from build123d import *

# Parameters (mm, degrees)
CROQUIS1_W              = 25
CROQUIS1_H              = 23
SALIENTE_EXTRUIR1_DEPTH = 2
CROQUIS2_W              = 8.5
CROQUIS2_H              = 8.5
SALIENTE_EXTRUIR2_DEPTH = 3
CROQUIS3_R              = 3.75
SALIENTE_EXTRUIR3_DEPTH = 3
CROQUIS4_R              = 0.875
CORTAR_EXTRUIR1_DEPTH   = 3
CROQUIS5_W              = 22
CROQUIS5_H              = 5.5
SALIENTE_EXTRUIR4_DEPTH = 2


with BuildPart() as part:
    # Croquis1 → Saliente-Extruir1 (new body)
    with BuildSketch(Plane(origin=(0, 0, 0), x_dir=(1, 0, 0), z_dir=(0, 1, 0))):
        Rectangle(CROQUIS1_W, CROQUIS1_H)
    extrude(amount=SALIENTE_EXTRUIR1_DEPTH)

    # Croquis2 → Saliente-Extruir2 (add)
    with BuildSketch(Plane.XZ):
        with Locations((0, -1.75)):
            Rectangle(CROQUIS2_W, CROQUIS2_H)
    extrude(amount=SALIENTE_EXTRUIR2_DEPTH)

    # Croquis3 → Saliente-Extruir3 (add)
    with BuildSketch(Plane.XZ.offset(3)):
        with Locations((0, -1.75)):
            Circle(CROQUIS3_R)
    extrude(amount=SALIENTE_EXTRUIR3_DEPTH)

    # Croquis4 → Cortar-Extruir1 (cut)
    with BuildSketch(Plane.XZ):
        with Locations((-10.625, 9.625)):
            Circle(CROQUIS4_R)
        with Locations((10.825, 9.625)):
            Circle(CROQUIS4_R)
        with Locations((10.825, -3.375)):
            Circle(CROQUIS4_R)
        with Locations((-10.625, -3.375)):
            Circle(CROQUIS4_R)
    extrude(amount=-CORTAR_EXTRUIR1_DEPTH, mode=Mode.SUBTRACT)

    # Croquis5 → Saliente-Extruir4 (add)
    with BuildSketch(Plane(origin=(0, 2, 0), x_dir=(1, 0, 0), z_dir=(0, 1, 0))):
        with Locations((0, 9.75)):
            Rectangle(CROQUIS5_W, CROQUIS5_H)
    extrude(amount=SALIENTE_EXTRUIR4_DEPTH)


solid = part.part
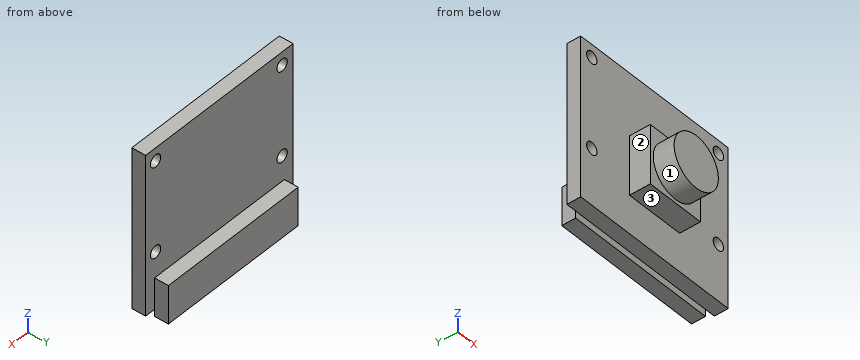
Model file for the job. Use its own axes, mm. Face numbers are marked on the shaded views. A direction names the side the tool comes from. Give positions to 0.01 mm unless a question says otherwise; leave off trailing zeros. Loops run counter-clockwise (first coordinate to the right, second up) from the corner with the lowest first, then second, coordinate; pieces in that order, holes last.
1) Wall check: line 1 (X direction, y = 1.25, z = -3); line 2 (Z direction, x = -6, y = 2.5); line 3 (Y direction, x = -3, z = 9). Give the ranges that are in metal, low to high.
2) Saw through at B-B (y = 0.75). Write the cut outline in (x, z) (3 decimals), plus the area to 3 significant figures.
3) Saw through at C-C (x = 0). Write the cut outline in (y, z).
4) Tool access for the marked faces 1, 2 and 3: list every direction of +Z, -Z, +X, -X, +Y, -Y with a clear straight run to the whole face (end or side of a thin tool).
5) Flat gauge pins, fed straight in: pin 1 Ø1.6 at (x, z) = (-10.625, -3.375) entering from -Y; pin 2 Ø3 at (x, z) = (10.825, 9.625) entering from -Y; pin 3 Ø0.9 at (x, y) = (-0.5, -1) entering from -Z; pin 4 Ø0.6 at (x, y) = (5, 1.5) entering from -Z. Where does each tip first touch, or does it go through?
6) Saw through at D-D (y = 2.5). Write the cut outline in (x, z).
7) Saw through at A-A (z = -1.75). Write the cut outline in (x, y), plus the area to 3 significant figures.
Answer block:
1. line 1: x = -12.5 to -11.42, -9.83 to 10.03, 11.62 to 12.5
1. line 2: z = -12.5 to -7
1. line 3: y = 0 to 2
2. outline: (-12.5, -11.5) - (12.5, -11.5) - (12.5, 11.5) - (-12.5, 11.5) - close; hole circle Ø1.75 at (-10.625, -3.375); hole circle Ø1.75 at (-10.625, 9.625); hole circle Ø1.75 at (10.825, -3.375); hole circle Ø1.75 at (10.825, 9.625)
2. area: 565 mm2
3. outline: (-6, -5.5) - (-3, -5.5) - (-3, -6) - (0, -6) - (0, -11.5) - (2, -11.5) - (2, -12.5) - (4, -12.5) - (4, -7) - (2, -7) - (2, 11.5) - (0, 11.5) - (0, 2.5) - (-3, 2.5) - (-3, 2) - (-6, 2) - close
4. face 1: -Y
4. face 2: +Z, -Z, -X, -Y
4. face 3: -Z, +X, -X, -Y
5. pin 1: passes through
5. pin 2: stops at y = 0
5. pin 3: stops at z = -6
5. pin 4: stops at z = -11.5
6. outline: (-11, -12.5) - (11, -12.5) - (11, -7) - (-11, -7) - close
7. outline: (-12.5, 0) - (-4.25, 0) - (-4.25, -3) - (-3.75, -3) - (-3.75, -6) - (3.75, -6) - (3.75, -3) - (4.25, -3) - (4.25, 0) - (12.5, 0) - (12.5, 2) - (-12.5, 2) - close
7. area: 98.0 mm2
